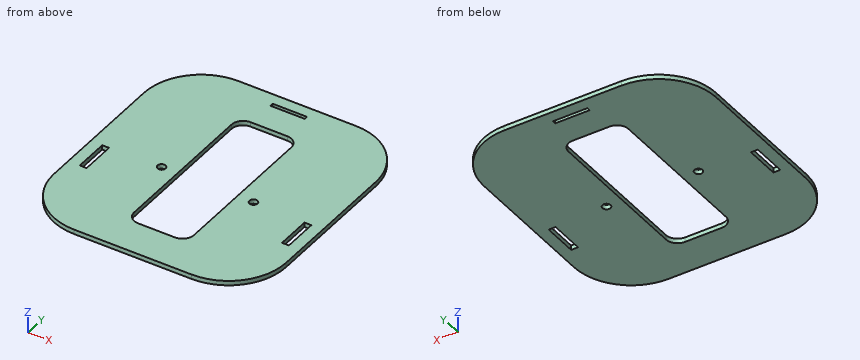
from build123d import *

# Parameters (mm, degrees)
SKETCH1_W           = 101
SKETCH1_H           = 110
BOSS_EXTRUDE1_DEPTH = 2
SKETCH3_W           = 15
SKETCH3_H           = 1.5
SKETCH3_W_2         = 3
SKETCH3_H_2         = 15
CUT_EXTRUDE1_DEPTH  = 128.433943673
FILLET2_R           = 25
SKETCH9_W           = 26
SKETCH9_H           = 75
CUT_EXTRUDE2_DEPTH  = 128.433943673
FILLET3_R           = 5
SKETCH4_R           = 1.75
CUT_EXTRUDE3_DEPTH  = 10


with BuildPart() as part:
    # Sketch1 → Boss-Extrude1 (new body)
    with BuildSketch(Plane.XY):
        with Locations((42.5, 32.1)):
            Rectangle(SKETCH1_W, SKETCH1_H)
    extrude(amount=BOSS_EXTRUDE1_DEPTH)

    # Sketch3 → Cut-Extrude1 (cut, through all)
    with BuildSketch(Plane.XY.offset(2)):
        with Locations((42.5, 81.35)):
            Rectangle(SKETCH3_W, SKETCH3_H)
        with Locations((-1.5, 19.1)):
            Rectangle(SKETCH3_W_2, SKETCH3_H_2)
        with Locations((86.5, 19.1)):
            Rectangle(SKETCH3_W_2, SKETCH3_H_2)
    extrude(amount=-CUT_EXTRUDE1_DEPTH, mode=Mode.SUBTRACT)

    # Fillet2
    fillet2_edges = [part.edges().sort_by_distance(p)[0] for p in [
        (-8, 87.1, 1),
        (93, 87.1, 1),
        (93, -22.9, 1),
        (-8, -22.9, 1),
    ]]
    fillet(fillet2_edges, radius=FILLET2_R)

    # Sketch9 → Cut-Extrude2 (cut, through all)
    with BuildSketch(Plane.XY.offset(2)):
        with Locations((42.5, 30.6)):
            Rectangle(SKETCH9_W, SKETCH9_H)
    extrude(amount=-CUT_EXTRUDE2_DEPTH, mode=Mode.SUBTRACT)

    # Fillet3
    fillet3_edges = [part.edges().sort_by_distance(p)[0] for p in [
        (29.5, -6.9, 1),
        (29.5, 68.1, 1),
        (55.5, 68.1, 1),
        (55.5, -6.9, 1),
    ]]
    fillet(fillet3_edges, radius=FILLET3_R)

    # Sketch4 → Cut-Extrude3 (cut)
    with BuildSketch(Plane.XY.offset(2)):
        with Locations((22.5, 27.1)):
            Circle(SKETCH4_R)
        with Locations((62.5, 27.1)):
            Circle(SKETCH4_R)
    extrude(amount=-CUT_EXTRUDE3_DEPTH, mode=Mode.SUBTRACT)


solid = part.part
For this review, take the finished solid that the model builds, in its own axes (mm). Give positions to 0.01 mm unless a question says otherwise; leave off trailing zeros. Order: outer loops, then holes, each group sorted by start corner. A loop starts at its lowest first (then second) coordinate and runs counter-clockwise, first axis right, second up. Notation, with made-up numbers: (59.5, 74) - (85.5, 74) arc R25 cw to (85.5, 99) - close; hole circle Ø9 at (62.5, -31). An arc over 180 degrees is marked (long way). Answer as a JSON object with one key per item and string values. Group by question number.
Item 1: Wall thickness on line 1 along Y through (x, z) = (40, 1.35); line 2 along X through (y, z) = (37, 0.9); line 3 along Y through (x, z) = (62.5, 1.25): over which ranges is each line inside the solid? List them lowest first.
Item 2: Take a section at B-B on y = 45.5. Give the boundary of the cut face in (x, z).
Item 3: Take a section at A-A on z = 1.4. Give the number of separate pieces and of enclosed holes in the cut face, and give its area (3 significant figures).
Item 4: Take a section at C-C on x = 22.5. Give the boundary of the cut face in (y, z).
Item 5: Clearance check with flat-ended pins moving along their axes: pin 1 Ø0.8 at (y, z) = (81.5, 0.5) entering from -X; pin 2 Ø1 at (x, z) = (-1.5, 1.5) entering from +Y. State where each tip first meets the part, or that it passes through.
Item 6: Take a section at D-D on x = 38. Give the boundary of the cut face in (y, z).
Reported:
{
 "1": {"line 1": "-22.9 to -6.9, 68.1 to 80.6, 82.1 to 87.1", "line 2": "-8 to 29.5, 55.5 to 93", "line 3": "-22.9 to 25.35, 28.85 to 87.1"},
 "2": {"outline": "(-8, 0) - (29.5, 0) - (29.5, 2) - (-8, 2) - close; (55.5, 0) - (93, 0) - (93, 2) - (55.5, 2) - close"},
 "3": {"separate pieces": "1", "enclosed holes": "6", "area": "8,510 mm^2"},
 "4": {"outline": "(-22.9, 0) - (25.35, 0) - (25.35, 2) - (-22.9, 2) - close; (28.85, 0) - (87.1, 0) - (87.1, 2) - (28.85, 2) - close"},
 "5": {"pin 1": "x = 0.75", "pin 2": "y = 79.45"},
 "6": {"outline": "(-22.9, 0) - (-6.9, 0) - (-6.9, 2) - (-22.9, 2) - close; (68.1, 0) - (80.6, 0) - (80.6, 2) - (68.1, 2) - close; (82.1, 0) - (87.1, 0) - (87.1, 2) - (82.1, 2) - close"}
}
